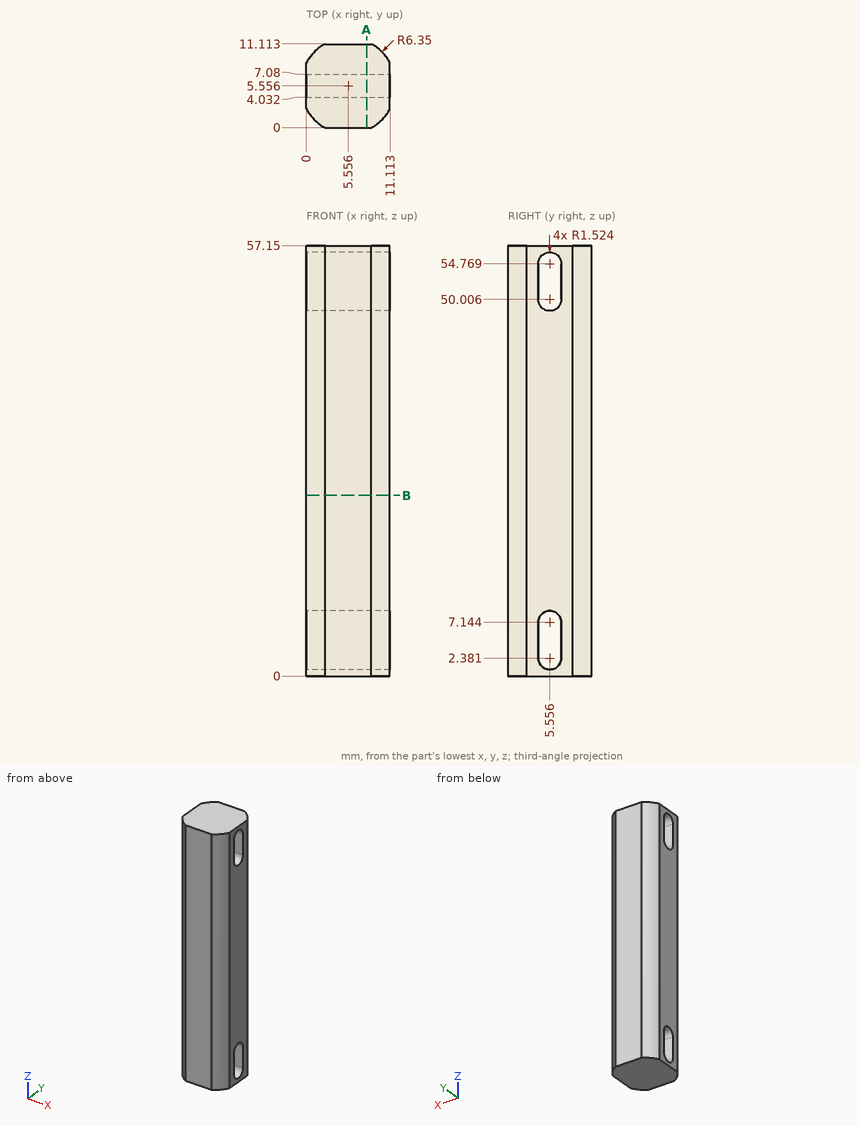
Geometry check sheet. Reference: drawing and pictorial views, mm from the part's lowest x, y, z. Give positions to 0.01 mm unless a question says otherwise; leave off trailing zeros. Order: outer loops, then holes, each group sorted by start corner. A loop starts at its lowest first (then second) coordinate and runs counter-clockwise, first axis right, second up.
1. Section check A-A, the plane x = 8. Give the number of separate pieces and of enclosed holes in the cut face.
2. Thickness scan on L1, parallel to Y at x = 6, z = 52.5; L2, parallel to Y at x = 2.25, z = 49 (1 decimal); L3, parallel to X at y = 1.75, z = 18 (1 decimal). Record the ranges inside material, lowest first.
3. Gauge pin test, flat end, axial feed: pin 1 Ø1.5 at (x, z) = (9, 47) entering from -Y. Record the tip position at first contact, or that the pin passes through.
4. Section check B-B, the plane z = 24. Enter the section's corners in (x, y), and give its area (4 significant figures).
Values follow:
1. separate pieces: 1
1. enclosed holes: 2
2. L1: y = 0 to 4.03, 7.08 to 11.11
2. L2: y = 0.1 to 4.4, 6.7 to 11
2. L3: x = 0.5 to 10.6
3. pin 1: stops at y = 0
4. outline: (0, 2.48) arc R6.35 ccw to (2.48, 0) - (8.63, 0) arc R6.35 ccw to (11.11, 2.48) - (11.11, 8.63) arc R6.35 ccw to (8.63, 11.11) - (2.48, 11.11) arc R6.35 ccw to (0, 8.63) - close
4. area: 113.5 mm2
